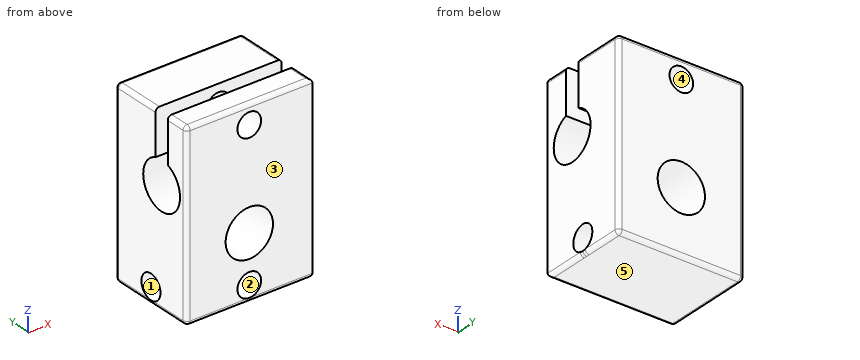
Autodesk Inventor part; units mm, degrees
ref_plane "YZ Plane" through (0, 0, 0) normal (1, 0, 0) x (0, 1, 0)
ref_plane "XZ Plane" through (0, 0, 0) normal (0, 1, 0) x (-1, 0, 0)
ref_plane "XY Plane" through (0, 0, 0) normal (0, 0, 1) x (1, 0, 0)
sketch "Sketch1" plane through (0, 0, 0) normal (0, 1, 0) x (-1, 0, 0)
  line L0 (-8, 11.5) -> (8, 11.5)
  line L1 (8, 11.5) -> (8, -11.5)
  line L2 (8, -11.5) -> (-8, -11.5)
  line L3 (-8, -11.5) -> (-8, 11.5)
  line L4 (-8, 11.5) -> (8, -11.5) construction
  line L5 (8, 11.5) -> (-8, -11.5) construction
  point P0 (0, 0)
  dimension "d0" = 16
  dimension "d1" = 23
extrude "Extrusion1" add sketch "Sketch1" along normal blind 11.5
sketch "Sketch2" plane through (8, 0, 11.5) normal (1, 0, 0) x (0, 0, -1)
  arc A0 (5.6716, 3) -> (5.6716, 5) centre (8.5, 4) ccw
  line L0 (23, 0) -> (23, 11.5)
  line L1 (23, 0) -> (0, 0)
  line L2 (0, 5) -> (5.6716, 5)
  line L3 (0, 5) -> (0, 3)
  line L4 (0, 0) -> (0, 11.5)
  line L5 (0, 3) -> (5.6716, 3)
  line L6 (8.5, 4) -> (0, 4) construction
  circle A1 centre (21, 5.74) radius 1.55
  point P0 (11.5, 0)
  dimension "d4" = 14.5
  dimension "d5" = 6
  dimension "d6" = 4
  dimension "d7" = 8.5
  dimension "d8" = 2
  dimension "d9" = 3.1
  dimension "d10" = 2
  dimension "d11" = 5.74
extrude "Extrusion2" cut sketch "Sketch2" against normal through all
sketch "Sketch3" plane through (0, 11.5, 0) normal (0, 1, 0) x (1, 0, 0)
  line L0 (8, -11.5) -> (-8, -11.5) construction
  line L1 (0, -11.5) -> (0, 11.545) construction
  circle A0 centre (0, 3.5) radius 3
  circle A1 centre (0, -9) radius 1.5
  line L2 (8, 11.5) -> (-8, 11.5)
  point P0 (0, 0)
  dimension "d14" = 8
  dimension "d15" = 6
  dimension "d17" = 20.5
  dimension "d18" = 3
extrude "Extrusion3" cut sketch "Sketch3" against normal through all
sketch "Sketch4" plane through (0, 0, 0) normal (0, -1, 0) x (1, 0, 0)
  line L0 (0, 0) -> (0, -11.4648) construction
  circle A0 centre (0, -9.5) radius 1.5
  line L1 (-8, -11.5) -> (8, -11.5)
  dimension "d21" = 3
  dimension "d22" = 2
extrude "Extrusion4" cut sketch "Sketch4" against normal up to surface
fillet "Fillet1" radius 0.5 13 edges at (8, 11.5, 0) (8, 5.75, -11.5) (-8, 5.75, -11.5) (0, 11.5, -11.5) (0, 0, -11.5) (-8, 0, 0) (-8, 11.5, 0) (8, 8.25, 11.5) (8, 1.5, 11.5) (-8, 1.5, 11.5) (-8, 8.25, 11.5) (0, 11.5, 11.5) (0, 0, 11.5)
thread "Thread1"
thread "Thread2"
thread "Thread3"
thread "Thread4"
properties part number "E3Dv6_Heater_Block"
Build history of the part. All positions in model axes, mm. Face numbers are marked on the shaded views. A direction names the side the tool comes from. Round coordinates to 2 decimals unless told otherwise and drop trailing zeros. Order: outer loops, then holes, each group sorted by start corner. A loop starts at its lowest first (then second) coordinate and runs counter-clockwise, first axis right, second up. Notation, with made-up numbers: (-34.75, 61.5) -> (4.25, 61.5) arc R23 cw to (4.25, 75.5) -> close; hole circle Ø10 at (9.5, -35). An arc over 180 degrees is marked (long way). Answer in a Markdown table with one row per item.
1) Band-saw the part on C-C on y = 10. Give the cut face in (x, z), and give its area (3 significant figures).
Values:
| item | result |
|---|---|
| outline | (-8, -11) arc R0.5 ccw to (-7.5, -11.5) -> (7.5, -11.5) arc R0.5 ccw to (8, -11) -> (8, 11) arc R0.5 ccw to (7.5, 11.5) -> (-7.5, 11.5) arc R0.5 ccw to (-8, 11) -> close; hole circle Ø6 at (0, -3.5); hole circle Ø3 at (0, 9) |
| area | 332 mm2 |
2) Band-saw the part on D-D on z = -9.5. Give the cut face in (x, y).
Values:
| item | result |
|---|---|
| outline | (-8, 0.5) arc R0.5 ccw to (-7.5, 0) -> (-1.5, 0) -> (-1.5, 4.19) -> (-8, 4.19) -> close; (-8, 7.29) -> (8, 7.29) -> (8, 11) arc R0.5 ccw to (7.5, 11.5) -> (-7.5, 11.5) arc R0.5 ccw to (-8, 11) -> close; (1.5, 0) -> (8, 0) -> (8, 4.19) -> (1.5, 4.19) -> close |
3) Band-saw the part on B-B on x = 2. Give the cut face in (y, z).
Values:
| item | result |
|---|---|
| outline | (0, -11) arc R0.5 ccw to (0.5, -11.5) -> (11, -11.5) arc R0.5 ccw to (11.5, -11) -> (11.5, -5.74) -> (0, -5.74) -> close; (0, -1.26) -> (11.5, -1.26) -> (11.5, 11) arc R0.5 ccw to (11, 11.5) -> (5, 11.5) -> (5, 5.83) arc R3 cw (long way) to (3, 5.83) -> (3, 11.5) -> (0.5, 11.5) arc R0.5 ccw to (0, 11) -> close; hole circle Ø3.1 at (5.74, -9.5) |
4) Band-saw the part on A-A on y = 2.5. Give the cut face in (x, z).
Values:
| item | result |
|---|---|
| outline | (-8, -11) arc R0.5 ccw to (-7.5, -11.5) -> (7.5, -11.5) arc R0.5 ccw to (8, -11) -> (8, 0.4) -> (-8, 0.4) -> close; (-8, 5.6) -> (8, 5.6) -> (8, 11) arc R0.5 ccw to (7.5, 11.5) -> (-7.5, 11.5) arc R0.5 ccw to (-8, 11) -> close; hole circle Ø6 at (0, -3.5); hole circle Ø3 at (0, -9.5); hole circle Ø3 at (0, 9) |
5) Mould opens along Z. For the marked faces 3, 4 and 5 say: released by +Z, released by -Z, zero draft, split by the parting line, or undercut.
Values:
| item | result |
|---|---|
| face 3 | zero draft |
| face 4 | undercut |
| face 5 | released by -Z |
6) Wall check: L1, parallel to X at y = 5, z = -3.5; L2, parallel to Z at x = 4.75, y = 6; L3, parallel to X at y = 1.45, z = 9. Give the ranges that are in metal, low to high.
Values:
| item | result |
|---|---|
| L1 | -8 to -3, 3 to 8 |
| L2 | -11.5 to -11.03, -7.97 to 0.76, 5.24 to 11.5 |
| L3 | -8 to -1.5, 1.5 to 8 |
7) Which spindle directions (+Z, -Z, +X, -X, +Y, -Y) get a long thin tool onto all of the face, cutting with end or side? Do the marked faces 1 and 2. Say none if no direction does.
Values:
| item | result |
|---|---|
| face 1 | +X, -X |
| face 2 | -Y |
8) Pin check, flat tip, straight feed: P1, Ø2.5, axis at x = 0, z = 9, coming from the -Y side. Stop position of the tip, or through.
Values:
| item | result |
|---|---|
| P1 | through |
